The listing builds one solid part. Answer for the finished solid, in the listing's coordinates (mm). Coordinates: 2 decimals unless noted, no trailing zeros. Order: outer loops, then holes, each group sorted by start corner. A loop starts at its lowest first (then second) coordinate and runs counter-clockwise, first axis right, second up. Notation, with made-up numbers: (81, -16) -> (98, -16) arc R10 cw to (98, -1) -> close; hole circle Ø5 at (-22.75, 77.5). An arc over 180 degrees is marked (long way). Return JSON: item names as keys, results as strings.
from build123d import *

# Parameters (mm, degrees)
BOSS_EXTRUDE2_DEPTH = 1
SKETCH6_R           = 0.75
CUT_EXTRUDE3_DEPTH  = 10


with BuildPart() as part:
    # Sketch4 → Boss-Extrude2 (new body)
    with BuildSketch(Plane(origin=(0, 0, 0), x_dir=(1, 0, 0), z_dir=(0, 1, 0))):
        with BuildLine():
            Line((-19.253709209, -12.655761176), (-13.682264454, -4.351605389))
            ThreePointArc((-13.682264454, -4.351605389), (-13.599577219, -4.243463868), (-13.518155162, -4.134366591))
            ThreePointArc((-13.518155162, -4.134366591), (-0.727323966, -7.891124567), (11.63634616, -2.905319296))
            ThreePointArc((11.63634616, -2.905319296), (0.692257999, -12.564498934), (-13.765160625, -14.578416434))
            ThreePointArc((-13.765160625, -14.578416434), (-16.57001445, -13.790023452), (-19.253709209, -12.655761176))
        make_face()
    extrude(amount=BOSS_EXTRUDE2_DEPTH)

    # Sketch6 → Cut-Extrude3 (cut)
    with BuildSketch(Plane(origin=(0, 1, 0), x_dir=(1, 0, 0), z_dir=(0, 1, 0))):
        with Locations((-12.937427019, -9.919909774)):
            Circle(SKETCH6_R)
    extrude(amount=-CUT_EXTRUDE3_DEPTH, mode=Mode.SUBTRACT)


solid = part.part
1. Consider line 1 (X direction, y = 0.75, z = 10.5); line 2 (X direction, y = 0.3, z = 5); line 3 (X direction, y = 0.05, z = 8). Determine where each line is inside the solid, lowest interval first. Write a range as from..to.
Answer block:
{"line 1": "x = -17.81..-13.41, -12.46..4.35", "line 2": "x = -14.12..-12.2, 8.76..10.19", "line 3": "x = -16.13..7.47"}
2. The part is cut by section C-C on z = 10.25. Give the vertices of the cut face in (x, y), and give its area (3 significant figures).
Answer block:
{"outline": "(-17.64, 0) -> (-13.61, 0) -> (-13.61, 1) -> (-17.64, 1) -> close; (-12.26, 0) -> (4.71, 0) -> (4.71, 1) -> (-12.26, 1) -> close", "area": "21.0 mm2"}
3. The part is cut by section D-D on x = 2.5. Give the vertices of the cut face in (y, z), and give its area (3 significant figures).
Answer block:
{"outline": "(0, 7.47) -> (1, 7.47) -> (1, 11.64) -> (0, 11.64) -> close", "area": "4.17 mm2"}
4. Determine the mould class of faces 1 (the face through (-13.687, 0.507, 9.887)), 2 (the face through (0.88, 0.493, 12.477)), 3 (the face through (-7, 1, 10)), 4 (the face through (-16.507, 0.493, 8.562)) for opening direction Z: pulls with the +Z half, pulls with the -Z half, needs draft (parallel to the pull), parting line crosses it, or undercut.
Answer block:
{"face 1": "undercut", "face 2": "pulls with the +Z half", "face 3": "needs draft", "face 4": "pulls with the -Z half"}
5. The part is cut by section A-A on z = 5.25. Give the vertices of the cut face in (x, y), and give its area (3 significant figures).
Answer block:
{"outline": "(-14.29, 0) -> (-11.77, 0) -> (-11.77, 1) -> (-14.29, 1) -> close; (8.34, 0) -> (9.99, 0) -> (9.99, 1) -> (8.34, 1) -> close", "area": "4.16 mm2"}
6. This flat-tipped pin is pushed along its axis until it touches: pin 1 Ø4 at (x, z) = (-14, 5.5) entering from -Y. Where does it stop, or does it pass through?
Answer block:
{"pin 1": "stops at y = 0"}
